from build123d import *

# Parameters (mm, degrees)
F0_W      = 65.8210366964
F0_H      = 53.360377121
F1_DEPTH  = 25.4
F0_W_2    = 8.4739662707
F2_DEPTH  = 16.256
F3_R      = 5.08
F4_R      = 5.08
F6_W      = 14.9103230797
F6_H      = 10.4163230571
F6_H_2    = 8.0820930889
F6_W_2    = 1.7418600619
F6_H_3    = 0.2754591405
F8_DEPTH  = 0.1778
F6_W_3    = 18.7708195299
F6_H_4    = 10.2186049917
F6_H_5    = 8.557209163
F6_W_4    = 1.9885748625
F9_DEPTH  = 0.2032
F10_W     = 1.7440356314
F10_H     = 0.2743424848
F11_DEPTH = 0.2032
F7_W      = 43.200377121
F7_H      = 4.064
F12_DEPTH = 66.04
F13_DEPTH = 14.986


# Not quite as in the source:
# - two fillets or chamfers of one size are made in one step


with BuildPart() as f1:
    # F0 (on Top) → F1 (new body)
    with BuildSketch(Plane.XY):
        Rectangle(F0_W, F0_H)
    extrude(amount=F1_DEPTH)

    # F0 (on Top) → F2 (join)
    with BuildSketch(Plane.XY):
        with Locations((-37.1475014836, 0)):
            Rectangle(F0_W_2, F0_H)
    extrude(amount=F2_DEPTH)

    # F3
    f3_edges = [f1.edges().sort_by_distance(p)[0] for p in [
        (-32.910518, 0, 25.4),
        (-41.384485, 0, 16.256),
    ]]
    fillet(f3_edges, radius=F3_R)

    # F4
    f4_edges = [f1.edges().sort_by_distance(p)[0] for p in [
        (2.54, -26.680189, 25.4),
        (2.54, 26.680189, 25.4),
        (32.910518, 0, 25.4),
        (-39.896587, -26.680189, 14.768102),
        (-39.896587, 26.680189, 14.768102),
        (-32.910518, -26.680189, 18.288),
        (-32.910518, 26.680189, 18.288),
        (-31.422621, -26.680189, 23.912102),
        (-34.607501, -26.680189, 16.256),
        (32.910518, -26.680189, 12.7),
        (-41.384485, -26.680189, 5.588),
        (-31.422621, 26.680189, 23.912102),
        (-34.607501, 26.680189, 16.256),
        (32.910518, 26.680189, 12.7),
        (-41.384485, 26.680189, 5.588),
    ]]
    fillet(f4_edges, radius=F4_R)

    # F6 (on face) → F8 (join)
    with BuildSketch(Plane.XZ.offset(26.6801885605)):
        Polygon((-19.7755768895, 0), (-4.168510437, 0), (-4.168510437, 11.176), (-4.168510437, 19.733209163), (-19.7755768895, 19.733209163), (-19.7755768895, 11.176), align=None)
        with Locations((-11.9322177488, 5.6890027045)):
            Rectangle(F6_W, F6_H, mode=Mode.SUBTRACT)
        with Locations((-11.9322177488, 15.2170465444)):
            Rectangle(F6_W, F6_H_2, mode=Mode.SUBTRACT)
        with Locations((-17.1627867967, 8.1434063613)):
            Rectangle(F6_W_2, F6_H_3)
    extrude(amount=F8_DEPTH)

    # F6 (on face) → F9 (join)
    with BuildSketch(Plane.XZ.offset(26.6801885605)):
        Polygon((8.2342270762, 20.32), (8.2342270762, 11.176), (8.2342270762, 0), (27.8305183482, 0), (27.8305183482, 11.176), (27.8305183482, 19.733209163), (27.8305183482, 20.32), align=None)
        with Locations((18.0146349594, 5.7878617372)):
            Rectangle(F6_W_3, F6_H_4, mode=Mode.SUBTRACT)
        with Locations((18.0146349594, 15.4546045815)):
            Rectangle(F6_W_3, F6_H_5, mode=Mode.SUBTRACT)
        with Locations((11.7142330855, 8.1434063613)):
            Rectangle(F6_W_4, F6_H_3)
    extrude(amount=F9_DEPTH)

    # F10 (on face) → F11 (join)
    with BuildSketch(Plane(origin=(0, 26.6801885605, 0), x_dir=(-1, 0, 0), z_dir=(0, 1, 0))):
        Polygon((-27.8305183482, 0), (-8.2305837423, 0), (-8.2305837423, 10.9018748626), (-8.2305837423, 20.32), (-27.8305183482, 20.32), (-27.8305183482, 11.2858796492), (-27.8305183482, 10.9018748626), align=None)
        Polygon((-8.626322262, 0.6852262607), (-27.4223405868, 0.7035561139), (-27.4223405868, 10.9018748626), (-8.626322262, 10.9018748626), align=None, mode=Mode.SUBTRACT)
        Polygon((-27.3978635669, 11.1784273759), (-27.3978635669, 19.7369996458), (-8.626322262, 19.7369996458), (-8.6272079498, 11.1749703065), align=None, mode=Mode.SUBTRACT)
        Polygon((-10.7196969911, 8.2838209346), (-12.7080604434, 8.287482895), (-12.7080604434, 8.0091850832), (-10.7196969911, 8.0091850832), align=None)
        Polygon((4.1694319807, 10.9128411859), (4.1694319807, 0), (19.7687353939, 0), (19.7687353939, 10.9128411859), (19.7687353939, 11.1958524212), (19.7687353939, 19.7498388588), (4.1547794826, 19.7498388588), (4.1547794826, 11.1958505586), align=None)
        Polygon((4.4739199802, 0.4796771973), (4.4739199802, 10.9128411859), (19.3859692663, 10.8820935711), (19.3859692663, 0.4796771973), align=None, mode=Mode.SUBTRACT)
        Polygon((19.3879064173, 19.2518327385), (19.3879064173, 11.1958524212), (4.4739199802, 11.1958505586), (4.4477242045, 19.2518327385), align=None, mode=Mode.SUBTRACT)
        with Locations((17.162848264, 8.1434589811)):
            Rectangle(F10_W, F10_H)
    extrude(amount=F11_DEPTH)

    # F7 (on face) → F12 (cut)
    with BuildSketch(Plane(origin=(-32.9105183482, 0, 0), x_dir=(0, -1, 0), z_dir=(-1, 0, 0))):
        with Locations((0, 18.288)):
            Rectangle(F7_W, F7_H)
    extrude(amount=-F12_DEPTH, mode=Mode.SUBTRACT)

    # F13 (cut): a face of the model
    f13_faces = [f1.faces().sort_by_distance(p)[0] for p in [
        (-1.6969831353, 0, 16.256),
    ]]
    extrude(f13_faces, amount=-F13_DEPTH, mode=Mode.SUBTRACT)


solid = f1.part
Verification items for the finished model (mm, model axes). A direction names the side the tool comes from. Give positions to 0.01 mm unless a question says otherwise; leave off trailing zeros. Write each loop counter-clockwise with the first axis right and the second up, starting at its lowest first coordinate (ties: lowest second). Pieces come first, ordered by that corner, then holes. Notation, with made-up numbers: (-14, -20) - (15, -20) arc R24 cw to (15, -9) - close; hole circle Ø8 at (83, -10). An arc over 180 degrees is marked (long way). Answer as CSV lines item,"result". Start each with the question number.
1. Sectioned sample at A-A (y = 10). Record the boundary of the cut face in (x, z), then the cut area to 3 significant figures.
2. Draft check along X on faces 5 (the face through (18, 26.68, 6)), 6 (the face through (-2, -21.6, 11)), 7 (the face through (-31.462, 0.302, 23.872)). Enter one of: pulls with the +X half, pulls with the -X half, needs draft (parallel to the pull), parting line crosses it, or undercut.
3. Sectioned sample at B-B (x = -24). Record the boundary of the cut face in (y, z), then the cut area to 3 significant figures.
4. Thickness scan on line 1 (Y direction, x = 12.5, z = 18.5); line 2 (Z direction, x = 19.5, y = 0); line 3 (Z direction, x = -36, y = -2.5). Record the ranges inside material, lowest first.
5. Depth check by flat-ended pin: pin 1 (6.5 mm diameter, centred on x = -12.5, z = 14.5, fed in from +Y); pin 2 (6 mm diameter, centred on x = -17, z = 9, fed in from -Y); pin 3 (10 mm diameter, centred on y = -13.5, z = 13.5, fed in from +X). Enter the tip coordinate at first touch or a pass-through.
6. Set-up check for faces 1 (the face through (-33.891, 25.729, 14.135)), 2 (the face through (-2, 0, 1.27)), 3 (the face through (-32.95, -25.793, 14.044)), 4 (the face through (-12, -26.68, 15)): record each of +Z, -Z, +X, -X, +Y, -Y from which the full face is reachable in a straight line by a thin tool's end or side.
Derived:
1,outline,"(-41.38, 0) - (32.91, 0) - (32.91, 1.27) - (-36.3, 1.27) - (-36.3, 16.26) arc R5.08 ccw to (-41.38, 11.18) - close; (-32.91, 20.32) - (32.91, 20.32) arc R5.08 ccw to (27.83, 25.4) - (-27.83, 25.4) arc R5.08 ccw to start"
1,area,"488 mm²"
2,face 5,"undercut"
2,face 6,"needs draft"
2,face 7,"pulls with the -X half"
3,outline,"(-26.68, 0) - (26.68, 0) - (26.68, 20.32) arc R5.08 ccw to (21.6, 25.4) - (-21.6, 25.4) arc R5.08 ccw to (-26.68, 20.32) - close; hole (-21.6, 1.27) - (21.6, 1.27) - (21.6, 20.32) - (-21.6, 20.32) - close"
3,area,"521 mm²"
4,line 1,"-26.68 to -21.6, 21.6 to 26.68"
4,line 2,"0 to 1.27, 20.32 to 25.4"
4,line 3,"0 to 1.27"
5,pin 1,"y = 26.68"
5,pin 2,"y = -26.86"
5,pin 3,"x = -36.3"
6,face 1,"+Z, -X, +Y"
6,face 2,"+X"
6,face 3,"+Z, -X, -Y"
6,face 4,"-Y"
